Autodesk Inventor part; units mm, degrees
ref_plane "YZ Plane" through (0, 0, 0) normal (1, 0, 0) x (0, 1, 0)
ref_plane "XZ Plane" through (0, 0, 0) normal (0, 1, 0) x (-1, 0, 0)
ref_plane "XY Plane" through (0, 0, 0) normal (0, 0, 1) x (1, 0, 0)
sketch "Sketch1" plane through (0, 0, 0) normal (0, 1, 0) x (-1, 0, 0)
  line L0 (0, 0) -> (0, -776.116)
  line L1 (-50, -734.6946) -> (-50, 0)
  line L2 (0, 0) -> (-173.6931, 0)
  line L3 (0, 0) -> (0, 776.116)
  line L4 (-50, 734.6946) -> (-50, 0)
  arc A0 (-106.066, 982.182) -> (-50, 734.6946) centre (0, 876.116) ccw
  arc A1 (-70.7107, 946.8267) -> (0, 776.116) centre (0, 876.116) ccw
  line L5 (-70.7107, 946.8267) -> (-106.066, 982.182)
  line L6 (0, -1268.9888) -> (0, 1481.1208) construction
  line L7 (0, -776.116) -> (0, -876.116)
  line L8 (0, -876.116) -> (-50, -876.116)
  line L9 (-50, -876.116) -> (-50, -734.6946)
  point P0 (0, -2.2081)
  point P1 (-13.1062, 0)
  point P2 (-20, -18.7767)
  point P3 (-20, 3.1509)
  point P4 (-46.6023, 0)
  point P5 (-20, -18.7767)
  dimension "d6" = 45
  dimension "d7" = 50
  dimension "d8" = 100
  dimension "d9" = 50
  dimension "d10" = 1752.232
revolve "Revolution1" add sketch "Sketch1" angle 360 about axis through (0, 0, -10) along (0, 0, 1)
sketch "Sketch2" plane through (0, 0, 0) normal (0, 1, 0) x (-1, 0, 0)
  line L0 (50, -876.116) -> (-50, -876.116)
  arc A0 (-100, -876.116) -> (100, -876.116) centre (0, -876.116) ccw
  line L1 (65.0556, -876.116) -> (-85.3956, -876.116)
  line L2 (0, -338.7665) -> (0, -580.5318)
  line L3 (100, -876.116) -> (100, -676.116)
  line L4 (100, -676.116) -> (-100, -676.116)
  line L5 (-100, -676.116) -> (-100, -876.116)
  point P0 (0, 0)
  dimension "d11" = 100
  dimension "d12" = 200
extrude "Extrusion1" add sketch "Sketch2" along normal mid plane 200
sketch "Sketch4" plane through (0, 0, 0) normal (0, 1, 0) x (-1, 0, 0)
  arc A0 (-100, -876.116) -> (100, -876.116) centre (0, -876.116) ccw construction
  circle A1 centre (0, -876.116) radius 50
  point P0 (0, 0)
  dimension "d16" = 50
extrude "Extrusion2" cut sketch "Sketch4" along normal through all both and the other way through all
sketch "Sketch6" plane through (0, 0, 0) normal (1, 0, 0) x (0, 1, 0)
  line L0 (-100, -976.116) -> (100, -976.116) construction
  line L1 (0, -623.7458) -> (0, -465.1617)
  line L2 (75, -976.116) -> (-75, -976.116)
  line L3 (-75, -976.116) -> (-75, -726.116)
  line L4 (-75, -726.116) -> (75, -726.116)
  line L5 (75, -726.116) -> (75, -976.116)
  point P0 (0, 0)
  point P1 (0, -976.116)
  dimension "d27" = 150
  dimension "d28" = 250
extrude "Extrusion4" cut sketch "Sketch6" along normal through all both and the other way through all
equation "\"d7\" = rod_radius"
equation "\"d8\" = S_radius"
equation "\"d9\" = rod_radius"
equation "\"d10\" = L1"
equation "\"d11\" = S_radius"
equation "\"d12\" = 2 * S_radius"
equation "\"d13\" = 2 * S_radius"
equation "\"d16\" = rod_radius"
equation "\"d27\" = 3 * rod_radius"
equation "\"d28\" = 5 * rod_radius"
equation "\"L1\" = 1752.23201"
equation "\"rod_radius\" = 50"
equation "\"S_radius\" = 2 * rod_radius"
equation "\"dyad1_Fx\" = -4260.66351"
equation "\"dyad1_Fy\" = 914.69194"
equation "\"dyad1_Fz\" = 2675.35545"
equation "\"dyad2_Fx\" = -451.87793"
equation "\"dyad2_Fy\" = -915.49296"
equation "\"dyad2_Fz\" = 3417.84038"
equation "\"dyad3_Fx\" = -4318"
equation "\"dyad3_Fz\" = 1248"
equation "\"dyad4_Fx\" = 2692.78997"
equation "\"dyad4_Fy\" = 2100.31348"
equation "\"dyad4_Fz\" = 2764.89028"
equation "\"dyad5_Fx\" = 3055.55556"
equation "\"dyad5_Fy\" = -2032.16374"
equation "\"dyad5_Fz\" = 2423.97661"
equation "\"L2\" = 1260.47471"
equation "\"L3\" = 1299.40028"
equation "\"L4\" = 3944.54642"
equation "\"L5\" = 2129.93938"
properties part number "US_Dyad-01"
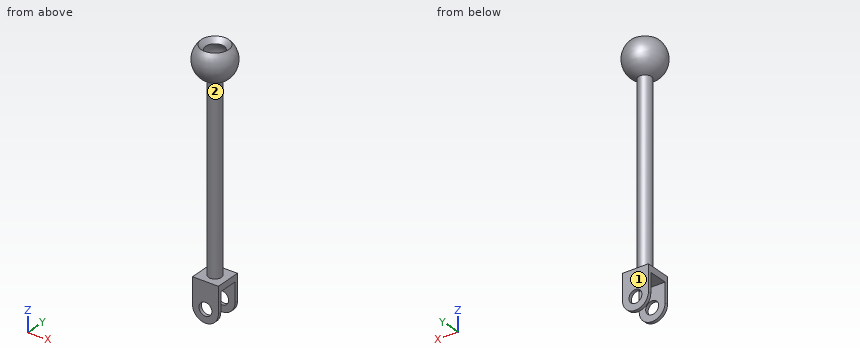
CAD build for the part. Positions are in the model's coordinates, mm. Face numbers are marked on the shaded views. Round coordinates to 2 decimals unless told otherwise and drop trailing zeros. Order: outer loops, then holes, each group sorted by start corner. A loop starts at its lowest first (then second) coordinate and runs counter-clockwise, first axis right, second up.
Q1. Slice it at B-B (z = -178). Write the cut outline in (x, y).
Q2. Two-plate mould, pull along Z, no slides. Class the marked faces 1 and 2: pulls with the +Z half, pulls with the -Z half, needs draft (parallel to the pull), parting line crosses it, or undercut.
Q3. Drop flat-ended pins along their axis: pin 1 (1.5 mm diameter, centred on y = -42.5, z = 635, fed in from +X); pin 2 (8 mm diameter, centred on x = 99.5, z = -676.5, fed in from -Y); pin 3 (8 mm diameter, centred on x = 69, y = -69.5, fed in from -Z). Give the stop position or say it passes through.
Q4. Slice it at A-A (x = 28). State how many separate pieces and enclosed holes the cut face has, and give its area (3 significant figures).
Q5. Wall check: L1, parallel to Z at x = -42.5, y = -80; L2, parallel to Z at x = 0, y = -82.75; L3, parallel to Y at x = 84.5, z = -861. Give the ranges that are in metal, low to high.
Results below:
1. outline: circle Ø100 at (0, 0)
2. face 1: needs draft
2. face 2: undercut
3. pin 1: stops at x = 27.51
3. pin 2: stops at y = -100
3. pin 3: stops at z = -726.12
4. separate pieces: 3
4. enclosed holes: 0
4. area: 165,000 mm2
5. L1: z = -966.64 to -902.46, -849.78 to -676.12, 756.56 to 833.76, 918.47 to 966.7
5. L2: z = -976.12 to -926.12, -826.12 to -676.12, 751.01 to 819.97, 932.26 to 958.87
5. L3: y = -100 to -75, 75 to 100
